Geometry check sheet. Reference: the model listing, model coordinates, mm. Coordinates: 2 decimals unless noted, no trailing zeros. Write each loop counter-clockwise with the first axis right and the second up, starting at its lowest first coordinate (ties: lowest second). Pieces come first, ordered by that corner, then holes. Notation, with made-up numbers: (10.25, -25) -> (29.25, -25) arc R30 ccw to (29.25, 7) -> close; hole circle Ø9 at (10.25, 44). An arc over 180 degrees is marked (long way). One line per question, with ' | ' between items.
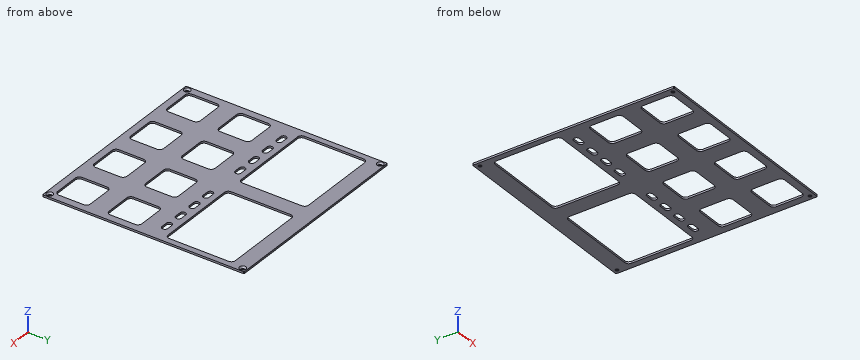
```python
from build123d import *

# Parameters (mm, degrees)
PAD_DEPTH        = 1
POCKET_DEPTH     = 0.001
HOLE_D           = 1.75
HOLE_CSINK_D     = 3.3
HOLE_CSINK_ANGLE = 90
POCKET008_DEPTH  = 1.001
POCKET010_DEPTH  = 5
POCKET011_DEPTH  = 1.001


with BuildPart() as part:
    # Sketch → Pad (new body)
    with BuildSketch(Plane.XY):
        with BuildLine():
            Line((-51.8, 52.175), (51.8, 52.175))
            ThreePointArc((52.175, 51.8), (52.065165, 52.065165), (51.8, 52.175))
            Line((52.175, 51.8), (52.175, -51.8))
            ThreePointArc((51.8, -52.175), (52.065165, -52.065165), (52.175, -51.8))
            Line((51.8, -52.175), (-51.8, -52.175))
            ThreePointArc((-52.175, -51.8), (-52.065165, -52.065165), (-51.8, -52.175))
            Line((-52.175, -51.8), (-52.175, 51.8))
            ThreePointArc((-51.8, 52.175), (-52.065165, 52.065165), (-52.175, 51.8))
        make_face()
    extrude(amount=-PAD_DEPTH)

    # Sketch002 → Pocket (cut, through all)
    with BuildSketch(Plane.XY.offset(-4.8)):
        with BuildLine():
            Line((-45, 50.175), (45, 50.175))
            ThreePointArc((45, 50.175), (45.353553, 50.321447), (45.5, 50.675))
            ThreePointArc((45.5, 50.675), (45.353553, 51.028553), (45, 51.175))
            Line((-45, 51.175), (45, 51.175))
            ThreePointArc((-45, 51.175), (-45.353553, 51.028553), (-45.5, 50.675))
            ThreePointArc((-45.5, 50.675), (-45.353553, 50.321447), (-45, 50.175))
        make_face()
        with BuildLine():
            Line((-45, -51.175), (45, -51.175))
            ThreePointArc((45, -51.175), (45.353553, -51.028553), (45.5, -50.675))
            ThreePointArc((45.5, -50.675), (45.353553, -50.321447), (45, -50.175))
            Line((-45, -50.175), (45, -50.175))
            ThreePointArc((-45, -50.175), (-45.353553, -50.321447), (-45.5, -50.675))
            ThreePointArc((-45.5, -50.675), (-45.353553, -51.028553), (-45, -51.175))
        make_face()
        with BuildLine():
            Line((51.175, -45), (51.175, 45))
            ThreePointArc((51.175, 45), (51.028553, 45.353553), (50.675, 45.5))
            ThreePointArc((50.675, 45.5), (50.321447, 45.353553), (50.175, 45))
            Line((50.175, -45), (50.175, 45))
            ThreePointArc((50.175, -45), (50.321447, -45.353553), (50.675, -45.5))
            ThreePointArc((50.675, -45.5), (51.028553, -45.353553), (51.175, -45))
        make_face()
        with BuildLine():
            Line((-50.175, -45), (-50.175, 45))
            ThreePointArc((-50.175, 45), (-50.321447, 45.353553), (-50.675, 45.5))
            ThreePointArc((-50.675, 45.5), (-51.028553, 45.353553), (-51.175, 45))
            Line((-51.175, -45), (-51.175, 45))
            ThreePointArc((-51.175, -45), (-51.028553, -45.353553), (-50.675, -45.5))
            ThreePointArc((-50.675, -45.5), (-50.321447, -45.353553), (-50.175, -45))
        make_face()
    extrude(amount=-POCKET_DEPTH, mode=Mode.SUBTRACT)

    # Hole (through all)
    with Locations(Plane.XY):
        with Locations((-50, 50), (50, 50), (50, -50), (-50, -50)):
            CounterSinkHole(HOLE_D / 2, HOLE_CSINK_D / 2, counter_sink_angle=HOLE_CSINK_ANGLE)

    # Sketch027 → Pocket008 (cut, through all)
    with BuildSketch(Plane.XY):
        with BuildLine():
            Line((-49.17, 11.27), (-49.17, 42.07))
            ThreePointArc((-47.17, 44.07), (-48.584214, 43.484214), (-49.17, 42.07))
            Line((-47.17, 44.07), (-6.17, 44.07))
            ThreePointArc((-4.17, 42.07), (-4.755786, 43.484214), (-6.17, 44.07))
            Line((-4.17, 42.07), (-4.17, 11.27))
            ThreePointArc((-6.17, 9.27), (-4.755786, 9.855786), (-4.17, 11.27))
            Line((-6.17, 9.27), (-47.17, 9.27))
            ThreePointArc((-49.17, 11.27), (-48.584214, 9.855786), (-47.17, 9.27))
        make_face()
        with BuildLine():
            Line((4.17, 11.27), (4.17, 42.07))
            ThreePointArc((6.17, 44.07), (4.755786, 43.484214), (4.17, 42.07))
            Line((6.17, 44.07), (47.17, 44.07))
            ThreePointArc((49.17, 42.07), (48.584214, 43.484214), (47.17, 44.07))
            Line((49.17, 42.07), (49.17, 11.27))
            ThreePointArc((47.17, 9.27), (48.584214, 9.855786), (49.17, 11.27))
            Line((47.17, 9.27), (6.17, 9.27))
            ThreePointArc((4.17, 11.27), (4.755786, 9.855786), (6.17, 9.27))
        make_face()
    extrude(amount=-POCKET008_DEPTH, mode=Mode.SUBTRACT)

    # Sketch029 → Pocket010 (cut)
    with BuildSketch(Plane.XY):
        with BuildLine():
            ThreePointArc((-33.17, 6.27), (-34.67, 4.77), (-33.17, 3.27))
            Line((-33.17, 3.27), (-30.17, 3.27))
            ThreePointArc((-30.17, 3.27), (-28.67, 4.77), (-30.17, 6.27))
            Line((-30.17, 6.27), (-33.17, 6.27))
        make_face()
        with BuildLine():
            ThreePointArc((-23.17, 6.27), (-24.67, 4.77), (-23.17, 3.27))
            Line((-23.17, 3.27), (-20.17, 3.27))
            ThreePointArc((-20.17, 3.27), (-18.67, 4.77), (-20.17, 6.27))
            Line((-20.17, 6.27), (-23.17, 6.27))
        make_face()
        with BuildLine():
            ThreePointArc((-13.17, 6.27), (-14.67, 4.77), (-13.17, 3.27))
            Line((-13.17, 3.27), (-10.17, 3.27))
            ThreePointArc((-10.17, 3.27), (-8.67, 4.77), (-10.17, 6.27))
            Line((-10.17, 6.27), (-13.17, 6.27))
        make_face()
        with BuildLine():
            ThreePointArc((-43.17, 6.27), (-44.67, 4.77), (-43.17, 3.27))
            Line((-43.17, 3.27), (-40.17, 3.27))
            ThreePointArc((-40.17, 3.27), (-38.67, 4.77), (-40.17, 6.27))
            Line((-40.17, 6.27), (-43.17, 6.27))
        make_face()
        with BuildLine():
            ThreePointArc((10.17, 6.27), (8.67, 4.77), (10.17, 3.27))
            Line((10.17, 3.27), (13.17, 3.27))
            ThreePointArc((13.17, 3.27), (14.67, 4.77), (13.17, 6.27))
            Line((13.17, 6.27), (10.17, 6.27))
        make_face()
        with BuildLine():
            ThreePointArc((20.17, 6.27), (18.67, 4.77), (20.17, 3.27))
            Line((20.17, 3.27), (23.17, 3.27))
            ThreePointArc((23.17, 3.27), (24.67, 4.77), (23.17, 6.27))
            Line((23.17, 6.27), (20.17, 6.27))
        make_face()
        with BuildLine():
            ThreePointArc((30.17, 6.27), (28.67, 4.77), (30.17, 3.27))
            Line((30.17, 3.27), (33.17, 3.27))
            ThreePointArc((33.17, 3.27), (34.67, 4.77), (33.17, 6.27))
            Line((33.17, 6.27), (30.17, 6.27))
        make_face()
        with BuildLine():
            ThreePointArc((40.17, 6.27), (38.67, 4.77), (40.17, 3.27))
            Line((40.17, 3.27), (43.17, 3.27))
            ThreePointArc((43.17, 3.27), (44.67, 4.77), (43.17, 6.27))
            Line((43.17, 6.27), (40.17, 6.27))
        make_face()
    extrude(amount=-POCKET010_DEPTH, mode=Mode.SUBTRACT)

    # Sketch030 → Pocket011 (cut, through all)
    with BuildSketch(Plane.XY):
        with BuildLine():
            Line((-48.505, -19.735), (-48.505, -6.935))
            ThreePointArc((-46.405, -4.835), (-47.889924, -5.450076), (-48.505, -6.935))
            Line((-46.405, -4.835), (-33.605, -4.835))
            ThreePointArc((-31.505, -6.935), (-32.120076, -5.450076), (-33.605, -4.835))
            Line((-31.505, -6.935), (-31.505, -19.735))
            ThreePointArc((-33.605, -21.835), (-32.120076, -21.219924), (-31.505, -19.735))
            Line((-33.605, -21.835), (-46.405, -21.835))
            ThreePointArc((-48.505, -19.735), (-47.889924, -21.219924), (-46.405, -21.835))
        make_face()
        with BuildLine():
            Line((-21.835, -19.735), (-21.835, -6.935))
            ThreePointArc((-19.735, -4.835), (-21.219924, -5.450076), (-21.835, -6.935))
            Line((-19.735, -4.835), (-6.935, -4.835))
            ThreePointArc((-4.835, -6.935), (-5.450076, -5.450076), (-6.935, -4.835))
            Line((-4.835, -6.935), (-4.835, -19.735))
            ThreePointArc((-6.935, -21.835), (-5.450076, -21.219924), (-4.835, -19.735))
            Line((-6.935, -21.835), (-19.735, -21.835))
            ThreePointArc((-21.835, -19.735), (-21.219924, -21.219924), (-19.735, -21.835))
        make_face()
        with BuildLine():
            Line((4.835, -19.735), (4.835, -6.935))
            ThreePointArc((6.935, -4.835), (5.450076, -5.450076), (4.835, -6.935))
            Line((6.935, -4.835), (19.735, -4.835))
            ThreePointArc((21.835, -6.935), (21.219924, -5.450076), (19.735, -4.835))
            Line((21.835, -6.935), (21.835, -19.735))
            ThreePointArc((19.735, -21.835), (21.219924, -21.219924), (21.835, -19.735))
            Line((19.735, -21.835), (6.935, -21.835))
            ThreePointArc((4.835, -19.735), (5.450076, -21.219924), (6.935, -21.835))
        make_face()
        with BuildLine():
            Line((31.505, -19.735), (31.505, -6.935))
            ThreePointArc((33.605, -4.835), (32.120076, -5.450076), (31.505, -6.935))
            Line((33.605, -4.835), (46.405, -4.835))
            ThreePointArc((48.505, -6.935), (47.889924, -5.450076), (46.405, -4.835))
            Line((48.505, -6.935), (48.505, -19.735))
            ThreePointArc((46.405, -21.835), (47.889924, -21.219924), (48.505, -19.735))
            Line((46.405, -21.835), (33.605, -21.835))
            ThreePointArc((31.505, -19.735), (32.120076, -21.219924), (33.605, -21.835))
        make_face()
        with BuildLine():
            Line((31.505, -46.405), (31.505, -33.605))
            ThreePointArc((33.605, -31.505), (32.120076, -32.120076), (31.505, -33.605))
            Line((33.605, -31.505), (46.405, -31.505))
            ThreePointArc((48.505, -33.605), (47.889924, -32.120076), (46.405, -31.505))
            Line((48.505, -33.605), (48.505, -46.405))
            ThreePointArc((46.405, -48.505), (47.889924, -47.889924), (48.505, -46.405))
            Line((46.405, -48.505), (33.605, -48.505))
            ThreePointArc((31.505, -46.405), (32.120076, -47.889924), (33.605, -48.505))
        make_face()
        with BuildLine():
            Line((4.835, -46.405), (4.835, -33.605))
            ThreePointArc((6.935, -31.505), (5.450076, -32.120076), (4.835, -33.605))
            Line((6.935, -31.505), (19.735, -31.505))
            ThreePointArc((21.835, -33.605), (21.219924, -32.120076), (19.735, -31.505))
            Line((21.835, -33.605), (21.835, -46.405))
            ThreePointArc((19.735, -48.505), (21.219924, -47.889924), (21.835, -46.405))
            Line((19.735, -48.505), (6.935, -48.505))
            ThreePointArc((4.835, -46.405), (5.450076, -47.889924), (6.935, -48.505))
        make_face()
        with BuildLine():
            Line((-21.835, -46.405), (-21.835, -33.605))
            ThreePointArc((-19.735, -31.505), (-21.219924, -32.120076), (-21.835, -33.605))
            Line((-19.735, -31.505), (-6.935, -31.505))
            ThreePointArc((-4.835, -33.605), (-5.450076, -32.120076), (-6.935, -31.505))
            Line((-4.835, -33.605), (-4.835, -46.405))
            ThreePointArc((-6.935, -48.505), (-5.450076, -47.889924), (-4.835, -46.405))
            Line((-6.935, -48.505), (-19.735, -48.505))
            ThreePointArc((-21.835, -46.405), (-21.219924, -47.889924), (-19.735, -48.505))
        make_face()
        with BuildLine():
            Line((-48.505, -46.405), (-48.505, -33.605))
            ThreePointArc((-46.405, -31.505), (-47.889924, -32.120076), (-48.505, -33.605))
            Line((-46.405, -31.505), (-33.605, -31.505))
            ThreePointArc((-31.505, -33.605), (-32.120076, -32.120076), (-33.605, -31.505))
            Line((-31.505, -33.605), (-31.505, -46.405))
            ThreePointArc((-33.605, -48.505), (-32.120076, -47.889924), (-31.505, -46.405))
            Line((-33.605, -48.505), (-46.405, -48.505))
            ThreePointArc((-48.505, -46.405), (-47.889924, -47.889924), (-46.405, -48.505))
        make_face()
    extrude(amount=-POCKET011_DEPTH, mode=Mode.SUBTRACT)


solid = part.part
```
(1) Material ranges on line 1 (X direction, y = 50, z = -0.8) (3 decimals); line 2 (X direction, y = 33, z = -0.1) (3 decimals), recorded low to high.
Answers below:
line 1: x = -52.175 to -50.875, -49.125 to 49.125, 50.875 to 52.175 | line 2: x = -52.175 to -49.17, -4.17 to 4.17, 49.17 to 52.175
(2) Cross-section at B-B (x = 27). Record the cut outline in (y, z) (3 decimals), plus the area to 4 significant figures.
Answers below:
outline: (-52.175, -1) -> (9.27, -1) -> (9.27, 0) -> (-52.175, 0) -> close; (44.07, -1) -> (52.175, -1) -> (52.175, 0) -> (44.07, 0) -> close | area: 69.55 mm²
(3) Depth check by flat-ended pin: P1, Ø1, axis at x = -3.5, y = 12, coming from the +Z side. Enter the tip coordinate at first touch or a pass-through.
Answers below:
P1: stops at z = 0
(4) Cross-section at A-A (y = 15). Record the cut outline in (x, z) (3 decimals), plus the area to 4 significant figures.
Answers below:
outline: (-52.175, -1) -> (-49.17, -1) -> (-49.17, 0) -> (-52.175, 0) -> close; (-4.17, -1) -> (4.17, -1) -> (4.17, 0) -> (-4.17, 0) -> close; (49.17, -1) -> (52.175, -1) -> (52.175, 0) -> (49.17, 0) -> close | area: 14.35 mm²
(5) Cross-section at C-C (z = -0.6). Count the separate pieces of the cut face and the enclosed holes in it, plus the area to 3 significant figures.
Answers below:
separate pieces: 1 | enclosed holes: 22 | area: 5,340 mm²
